The model under review builds one solid part; all positions refer to its coordinate system, in mm. A direction names the side the tool comes from. Coordinates: 2 decimals unless noted, no trailing zeros. Loops run counter-clockwise (first coordinate to the right, second up) from the corner with the lowest first, then second, coordinate; pieces in that order, holes last. Notation, with made-up numbers: M -5,84.5 L 32,84.5 A20 ccw 32,117.5 Z; hole C -36,42 d11. An arc over 180 degrees is marked long. Return JSON: item names as keys, results as strings.
```python
from build123d import *

# Parameters (mm, degrees)
SKETCH_1_W          = 36
SKETCH_1_H          = 16
EXTRUDE_1_DEPTH     = 2
EXTRUDE_2_DEPTH     = 2.9
SKETCH_3_W          = 4
SKETCH_3_H          = 6.2
EXTRUDE_3_DEPTH     = 8.8
SKETCH_4_W          = 8
SKETCH_4_H          = 10
EXTRUDE_4_DEPTH     = 5.9
SKETCH_5_R          = 1.75
CUT_EXTRUDE_1_DEPTH = 41.366322597


with BuildPart() as part:
    # Эскиз1 → Бобышка-Вытянуть1 (new body)
    with BuildSketch(Plane.XY):
        with Locations((18, -8)):
            Rectangle(SKETCH_1_W, SKETCH_1_H)
    extrude(amount=EXTRUDE_1_DEPTH)

    # Эскиз2 → Бобышка-Вытянуть2 (add)
    with BuildSketch(Plane.XY.offset(2)):
        with BuildLine():
            Line((3.25, -9.65), (22.75, -9.65))
            ThreePointArc((22.75, -9.65), (25.85, -12.75), (22.75, -15.85))
            Line((22.75, -15.85), (3.25, -15.85))
            ThreePointArc((3.25, -15.85), (0.15, -12.75), (3.25, -9.65))
        make_face()
    extrude(amount=EXTRUDE_2_DEPTH)

    # Эскиз3 → Бобышка-Вытянуть3 (add)
    with BuildSketch(Plane.XY.offset(4.9)):
        with Locations((8.5, -12.75)):
            Rectangle(SKETCH_3_W, SKETCH_3_H)
        with Locations((17.5, -12.75)):
            Rectangle(SKETCH_3_W, SKETCH_3_H)
    extrude(amount=EXTRUDE_3_DEPTH)

    # Эскиз4 → Бобышка-Вытянуть4 (add)
    with BuildSketch(Plane.XY.offset(2)):
        with Locations((31.75, -8)):
            Rectangle(SKETCH_4_W, SKETCH_4_H)
    extrude(amount=EXTRUDE_4_DEPTH)

    # Эскиз5 → Вырез-Вытянуть1 (cut, through all)
    with BuildSketch(Plane.XY.offset(4.9)):
        with Locations((3.25, -12.75)):
            Circle(SKETCH_5_R)
        with Locations((22.75, -12.75)):
            Circle(SKETCH_5_R)
    extrude(amount=-CUT_EXTRUDE_1_DEPTH, mode=Mode.SUBTRACT)


solid = part.part
```
1. Insertion check: pin 1 Ø2.5 at (x, y) = (12, -13.5) entering from +Z; pin 2 Ø1.9 at (y, z) = (-13, 11) entering from -X; pin 3 Ø1.9 at (y, z) = (-13, 8.5) entering from +X. Each pin has a flat end and moves straight along its axis. Give the tip position at first contact, or say it passes through.
Check values:
{"pin 1": "z = 4.9", "pin 2": "x = 6.5", "pin 3": "x = 35.75"}
2. To check wall thickness, follow line 1 (Y direction, x = 22.75, z = 3.4); line 2 (X direction, y = -9.75, z = 9); line 3 (X direction, y = -13.25, z = 1). State the ranges of each line that lie inside material, in increasing order.
Check values:
{"line 1": "-15.85 to -14.5, -11 to -9.65", "line 2": "6.5 to 10.5, 15.5 to 19.5", "line 3": "0 to 1.57, 4.93 to 21.07, 24.43 to 36"}
3. The part is to be moulded in two halves that separate along X. For faces 1 (the face through (32, -3, 5)), 2 (the face through (15.5, -13, 9)), 3 (the face through (0, -8, 1)), say which applies: released by +X, released by -X, zero draft, split by the parting line, or undercut.
Check values:
{"face 1": "zero draft", "face 2": "undercut", "face 3": "released by -X"}
4. Add section C-C on y = -4. Give the boundary of the cut face in (x, z).
Check values:
{"outline": "M 0,0 L 36,0 L 36,2 L 35.75,2 L 35.75,7.9 L 27.75,7.9 L 27.75,2 L 0,2 Z"}
5. Add section A-A on z = 10. Give the boundary of the cut face in (x, y), plus the area to 3 significant figures.
Check values:
{"outline": "M 6.5,-15.85 L 10.5,-15.85 L 10.5,-9.65 L 6.5,-9.65 Z; M 15.5,-15.85 L 19.5,-15.85 L 19.5,-9.65 L 15.5,-9.65 Z", "area": "49.6 mm²"}
6. Add section B-B on x = 29. Give the boundary of the cut face in (y, z), plus the area to 3 significant figures.
Check values:
{"outline": "M -16,0 L 0,0 L 0,2 L -3,2 L -3,7.9 L -13,7.9 L -13,2 L -16,2 Z", "area": "91.0 mm²"}
7. Machinability: for faces 4 (the face through (32, -13, 5)), 5 (the face through (27.75, -8, 5)), 6 (the face through (35.75, -8, 5)), 7 (the face through (6.5, -13, 9)), 8 (the face through (15, -9.65, 4)), which of the approach directions +Z, -Z, +X, -X, +Y, -Y give a long, thin tool a straight path to every point of the face, cutting with its end or side? Answer none if there is none.
Check values:
{"face 4": "+Z, +X, -Y", "face 5": "+Z, +Y, -Y", "face 6": "+Z, +X, +Y, -Y", "face 7": "+Z, -X, +Y, -Y", "face 8": "+Z, -X, +Y"}
